Design review of the part built by this model. Coordinates are the model's own, in mm. A direction names the side the tool comes from. Give positions to 0.01 mm unless a question says otherwise; leave off trailing zeros. Loops run counter-clockwise (first coordinate to the right, second up) from the corner with the lowest first, then second, coordinate; pieces in that order, holes last. Notation, with made-up numbers: (-29.5, 13.25) -> (7.5, 13.25) arc R20 cw to (7.5, 41.25) -> close; hole circle Ø8 at (5.5, 55). An arc over 180 degrees is marked (long way). Answer as CSV lines item,"result".
from build123d import *

# Parameters (mm, degrees)
SKETCH_8_W       = 25
SKETCH_8_H       = 25
SKETCH_8_W_2     = 4
SKETCH_8_H_2     = 21
SKETCH_8_W_3     = 2
EXTRUDE_7_DEPTH  = 25
SKETCH_9_W       = 25
SKETCH_9_H       = 25
EXTRUDE_8_DEPTH  = 2
SKETCH_14_W      = 25
SKETCH_14_H      = 1.5
EXTRUDE_11_DEPTH = 25
EXTRUDE_14_DEPTH = 6
EXTRUDE_16_DEPTH = 2


with BuildPart() as part:
    # 草图8 → 凸台-拉伸7 (new body)
    with BuildSketch(Plane.XY):
        Rectangle(SKETCH_8_W, SKETCH_8_H)
        with Locations((3.5, 0)):
            Rectangle(SKETCH_8_W_2, SKETCH_8_H_2, mode=Mode.SUBTRACT)
        with Locations((-3.5, 0)):
            Rectangle(SKETCH_8_W_2, SKETCH_8_H_2, mode=Mode.SUBTRACT)
        with Locations((-9.5, 0)):
            Rectangle(SKETCH_8_W_3, SKETCH_8_H_2, mode=Mode.SUBTRACT)
        with Locations((9.5, 0)):
            Rectangle(SKETCH_8_W_3, SKETCH_8_H_2, mode=Mode.SUBTRACT)
    extrude(amount=EXTRUDE_7_DEPTH)

    # 草图9 → 凸台-拉伸8 (add)
    with BuildSketch(Plane(origin=(0, 0, 0), x_dir=(-1, 0, 0), z_dir=(0, 0, -1))):
        Rectangle(SKETCH_9_W, SKETCH_9_H)
    extrude(amount=EXTRUDE_8_DEPTH)

    # 草图14 → 凸台-拉伸11 (add)
    with BuildSketch(Plane.XY.offset(25)):
        Rectangle(SKETCH_14_W, SKETCH_14_H)
        with Locations((0, 6)):
            Rectangle(SKETCH_14_W, SKETCH_14_H)
        with Locations((0, -6)):
            Rectangle(SKETCH_14_W, SKETCH_14_H)
    extrude(amount=-EXTRUDE_11_DEPTH)

    # 草图16 → 凸台-拉伸14 (add)
    with BuildSketch(Plane(origin=(0, 0, -2), x_dir=(-1, 0, 0), z_dir=(0, 0, -1))):
        Polygon((0, -12.5), (10.825317547, -6.25), (10.825317547, 6.25), (0, 12.5), (-10.825317547, 6.25), (-10.825317547, -6.25), align=None)
        Polygon((0, -10.190598923), (8.825317547, -5.095299462), (8.825317547, 5.095299462), (0, 10.190598923), (-8.825317547, 5.095299462), (-8.825317547, -5.095299462), align=None, mode=Mode.SUBTRACT)
    extrude(amount=EXTRUDE_14_DEPTH)

    # 草图18 → 凸台-拉伸16 (add)
    with BuildSketch(Plane(origin=(0, 0, -8), x_dir=(-1, 0, 0), z_dir=(0, 0, -1))):
        Polygon((0, 12.5), (-10.825317547, 6.25), (-10.825317547, -6.25), (0, -12.5), (10.825317547, -6.25), (10.825317547, 6.25), align=None)
    extrude(amount=EXTRUDE_16_DEPTH)


solid = part.part
Q1. The part is to be moulded in two halves that separate along Z. For faces 5 (the flat face through (-3, 9, 0)), 6 (the flat face through (4.35, 7.68, -4.96)), 7 (the flat face through (5.5, -9, 12)), say which applies: pulls with the +Z half, pulls with the -Z half, needs draft (parallel to the pull), parting line crosses it, or undercut.
Filled sheet:
face 5,"pulls with the +Z half"
face 6,"undercut"
face 7,"needs draft"
Q2. We need section C-C, the plane x = 9.75. State the section outline as (y, z) points.
Filled sheet:
outline,"(-12.5, -2) -> (-6.87, -2) -> (-6.87, -10) -> (6.87, -10) -> (6.87, -2) -> (12.5, -2) -> (12.5, 25) -> (10.5, 25) -> (10.5, 0) -> (6.75, 0) -> (6.75, 25) -> (5.25, 25) -> (5.25, 0) -> (0.75, 0) -> (0.75, 25) -> (-0.75, 25) -> (-0.75, 0) -> (-5.25, 0) -> (-5.25, 25) -> (-6.75, 25) -> (-6.75, 0) -> (-10.5, 0) -> (-10.5, 25) -> (-12.5, 25) -> close"
Q3. We need section A-A, the plane z = -2.5. State the section outline as (x, y) points.
Filled sheet:
outline,"(-10.83, -6.25) -> (0, -12.5) -> (10.83, -6.25) -> (10.83, 6.25) -> (0, 12.5) -> (-10.83, 6.25) -> close; hole (-8.83, -5.1) -> (0, -10.19) -> (8.83, -5.1) -> (8.83, 5.1) -> (0, 10.19) -> (-8.83, 5.1) -> close"
Q4. We need section B-B, the plane y = 2.5. State the section outline as (x, z) points, and give its area (3 significant figures).
Filled sheet:
outline,"(-12.5, -2) -> (-10.83, -2) -> (-10.83, -10) -> (10.83, -10) -> (10.83, -2) -> (12.5, -2) -> (12.5, 25) -> (10.5, 25) -> (10.5, 0) -> (8.5, 0) -> (8.5, 25) -> (5.5, 25) -> (5.5, 0) -> (1.5, 0) -> (1.5, 25) -> (-1.5, 25) -> (-1.5, 0) -> (-5.5, 0) -> (-5.5, 25) -> (-8.5, 25) -> (-8.5, 0) -> (-10.5, 0) -> (-10.5, 25) -> (-12.5, 25) -> close; hole (-8.83, -8) -> (8.83, -8) -> (8.83, -2) -> (-8.83, -2) -> close"
area,"442 mm^2"
Q5. For faces 1 (the flat face through (-3, 3, 0)), 2 (the flat face through (0, -12.5, 12)), 3 (the flat face through (-4.47, 7.61, -4.96)), 4 (the flat face through (-10.825, 0, -6)), list the 3-axis set-ups (+Z, -Z, +X, -X, +Y, -Y) from which the entire face can be reached by the end or side of a thin tool; tool diameter is ignored.
Filled sheet:
face 1,"+Z"
face 2,"+Z, -Z, +X, -X, -Y"
face 3,"none"
face 4,"-Z, -X, +Y, -Y"
Q6. We need section D-D, the plane x = 6.75. State the section outline as (y, z) points.
Filled sheet:
outline,"(-12.5, -2) -> (-8.6, -2) -> (-8.6, -10) -> (8.6, -10) -> (8.6, -2) -> (12.5, -2) -> (12.5, 25) -> (-12.5, 25) -> close; hole (-6.29, -8) -> (6.29, -8) -> (6.29, -2) -> (-6.29, -2) -> close"
Q7. To check wall thickness, follow probe 1 along Y at (x, z) = (5.25, 23); probe 2 along X at (y, z) = (-10, 7); probe 3 along Z at (x, y) = (0, 8.5). State the ranges of each line that lie inside material, in increasing order. Write a range as from..to.
Filled sheet:
probe 1,"y = -12.5..-10.5, -6.75..-5.25, -0.75..0.75, 5.25..6.75, 10.5..12.5"
probe 2,"x = -12.5..-10.5, -8.5..-5.5, -1.5..1.5, 5.5..8.5, 10.5..12.5"
probe 3,"z = -10..-8, -2..25"
